Could you check a few things on this model? Use its own coordinates, in mm. Face numbers are marked on the shaded views. A direction names the side the tool comes from. Round coordinates to 2 decimals unless told otherwise and drop trailing zeros. Write each loop counter-clockwise with the first axis right and the second up, starting at its lowest first coordinate (ties: lowest second). Pieces come first, ordered by that corner, then holes. Notation, with made-up numbers: (67, -38) -> (101, -38) arc R19 cw to (101, -27) -> close; hole circle Ø3 at (3.25, 5.5). An arc over 180 degrees is marked (long way). One line per question, with ' | ' between items. Start each with the question number.
1. Imagine slicing it at C-C, the plane y = 204. List the corners of the cut face in (x, z) for me, and give its area (3 significant figures).
2. Imagine slicing it at A-A, the plane x = -7.75. List the corners of the cut face in (y, z) for me, and give its area (3 significant figures).
3. For the marked faces 4 and 5, which set-ups out of +Z, -Z, +X, -X, +Y, -Y let a thin tool reach every point of the face, with its end or its side?
4. If I drill on line 1 along Y through (x, z) = (0, 13.05); line 2 along Y through (x, z) = (-12.35, 0); line 3 along X through (y, z) = (26, 9), over which ranges is the centre line in solid material (lowest first)? Write a range as [from, to].
5. Thinking about a two-plate mould opening in X: for the marked faces 1, 2 and 3, which applies, released by +X, released by -X, zero draft, split by the parting line, or undercut?
6. Imagine slicing it at B-B, the plane z = -8. List the corners of the cut face in (x, y) for me.
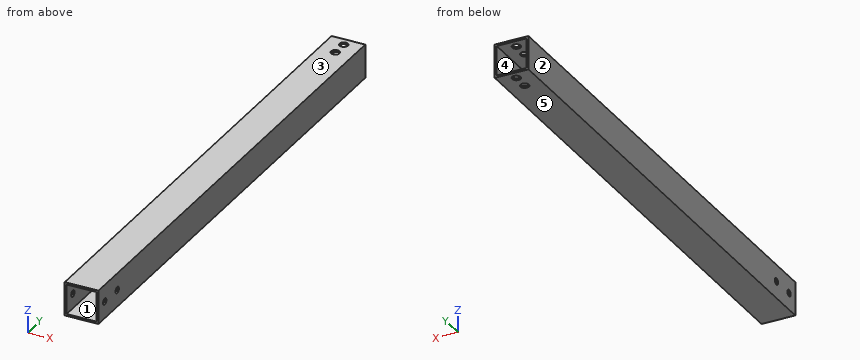
from build123d import *

# Parameters (mm, degrees)
SKETCH1_W               = 26.924
SKETCH1_H               = 26.924
SKETCH1_W_2             = 23.876
SKETCH1_H_2             = 23.876
EXTRUDE_THIN1_DEPTH     = 406.4
F_1_4_CLEARANCE_HOLE1_D = 6.7564
F_10_CLEARANCE_HOLE1_D  = 5.1054


with BuildPart() as part:
    # Sketch1 → Extrude-Thin1 (new body)
    with BuildSketch(Plane(origin=(0, 0, 0), x_dir=(1, 0, 0), z_dir=(0, 1, 0))):
        Rectangle(SKETCH1_W, SKETCH1_H)
        Rectangle(SKETCH1_W_2, SKETCH1_H_2, mode=Mode.SUBTRACT)
    extrude(amount=EXTRUDE_THIN1_DEPTH)

    # 1/4 Clearance Hole1 (through all)
    with Locations(Plane(origin=(0, 0, -13.462), x_dir=(-1, 0, 0), z_dir=(0, 0, -1))):
        with Locations((0, 399.2245), (0, 386.5245)):
            Hole(F_1_4_CLEARANCE_HOLE1_D / 2)

    # #10 Clearance Hole1 (through all)
    with Locations(Plane(origin=(13.462, 0, 0), x_dir=(0, 0, -1), z_dir=(1, 0, 0))):
        with Locations((0, 9.525), (0, 28.575)):
            Hole(F_10_CLEARANCE_HOLE1_D / 2)


solid = part.part
Geometry results:
1) outline: (-13.46, -13.46) -> (13.46, -13.46) -> (13.46, 13.46) -> (-13.46, 13.46) -> close; hole (-11.94, -11.94) -> (11.94, -11.94) -> (11.94, 11.94) -> (-11.94, 11.94) -> close | area: 155 mm2
2) outline: (0, -13.46) -> (406.4, -13.46) -> (406.4, -11.94) -> (0, -11.94) -> close; (0, 11.94) -> (406.4, 11.94) -> (406.4, 13.46) -> (0, 13.46) -> close | area: 1,240 mm2
3) face 4: +Y, -Y | face 5: -Z, +X, -X, +Y, -Y
4) line 1: y = [0, 383.15], [389.9, 395.85], [402.6, 406.4] | line 2: y = [0, 6.97], [12.08, 26.02], [31.13, 406.4] | line 3: x = [-13.46, -11.94], [11.94, 13.46]
5) face 1: undercut | face 2: released by -X | face 3: zero draft
6) outline: (-13.46, 0) -> (-11.94, 0) -> (-11.94, 406.4) -> (-13.46, 406.4) -> close; (11.94, 0) -> (13.46, 0) -> (13.46, 406.4) -> (11.94, 406.4) -> close
